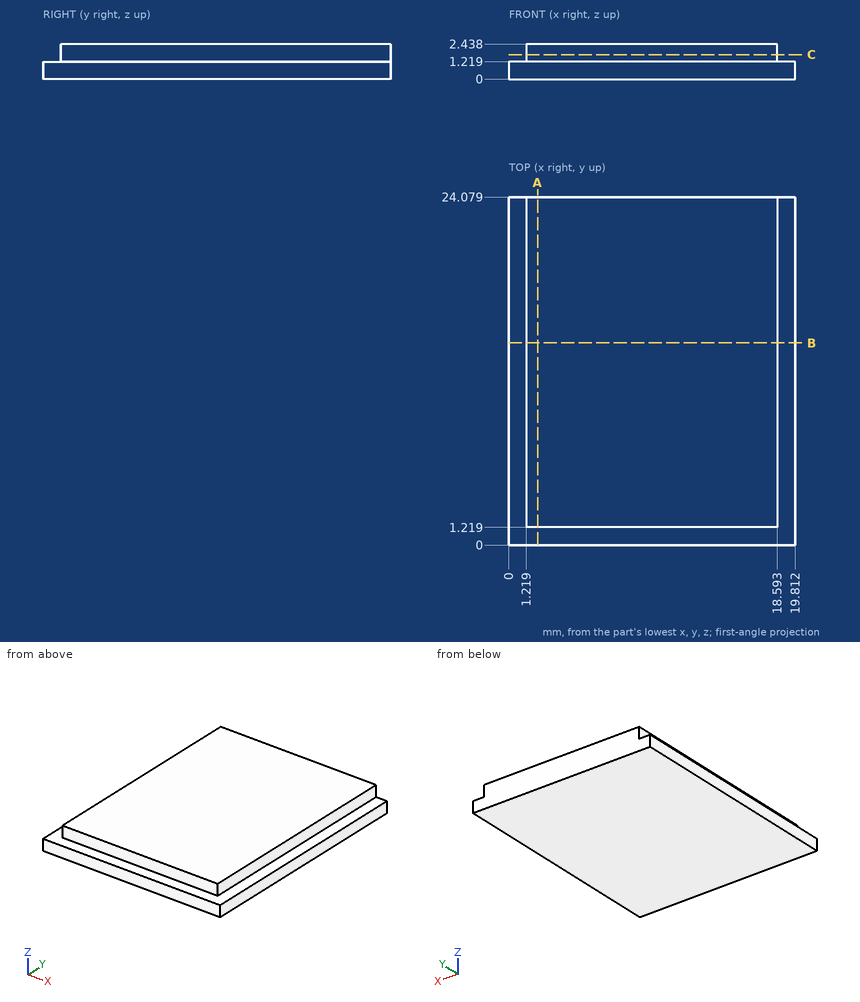
Study the drawing (mm; zero at the part's minimum x, y, z) and answer. Coordinates: 2 decimals unless noted, no trailing zeros. Write each loop counter-clockwise with the first axis right and the second up, starting at its lowest first coordinate (ties: lowest second). Pieces come first, ordered by that corner, then holes.
Q1. A cutting plane is placed at B-B, the plane y = 14. Give the vertices of the cut face in (x, z).
Q2. A cutting plane is placed at A-A, the plane x = 2. Give the vertices of the cut face in (y, z).
Q3. Find the intervals of material crossed by line 1 (Y direction, x = 1.75, z = 2.25); line 2 (X direction, y = 20.5, z = 2.15), in increasing order.
Q4. A cutting plane is placed at C-C, the plane z = 1.7. Give the vertices of the cut face in (x, y).
Findings below:
1. outline: (0, 0) - (19.81, 0) - (19.81, 1.22) - (18.59, 1.22) - (18.59, 2.44) - (1.22, 2.44) - (1.22, 1.22) - (0, 1.22) - close
2. outline: (0, 0) - (24.08, 0) - (24.08, 2.44) - (1.22, 2.44) - (1.22, 1.22) - (0, 1.22) - close
3. line 1: y = 1.22 to 24.08
3. line 2: x = 1.22 to 18.59
4. outline: (1.22, 1.22) - (18.59, 1.22) - (18.59, 24.08) - (1.22, 24.08) - close
